from build123d import *

# Parameters (mm, degrees)
BOSS_EXTRUDE1_DEPTH = 3.175
FILLET1_R           = 25.4
SKETCH2_R           = 2.25
CUT_EXTRUDE1_DEPTH  = 94.20730796


with BuildPart() as part:
    # Sketch1 → Boss-Extrude1 (new body)
    with BuildSketch(Plane.XY):
        with BuildLine():
            Line((-14.497184722, -4.405622253), (80.752815278, -4.405622253))
            Line((80.752815278, -4.405622253), (80.752815278, -38.596437465))
            ThreePointArc((80.752815278, -38.596437465), (66.572735919, -34.398241716), (57.985570414, -46.438178872))
            Line((57.985570414, -46.438178872), (-14.497184722, -46.438178872))
            Line((-14.497184722, -46.438178872), (-14.497184722, -4.405622253))
        make_face()
        with BuildLine():
            Line((8.180129042, -20.254648783), (43.838119696, -20.254648783))
            ThreePointArc((43.838119696, -20.254648783), (49.538039085, -25.954568173), (43.838119696, -31.654487563))
            Line((43.838119696, -31.654487563), (8.180129042, -31.654487563))
            ThreePointArc((8.180129042, -31.654487563), (2.480209652, -25.954568173), (8.180129042, -20.254648783))
        make_face(mode=Mode.SUBTRACT)
    extrude(amount=BOSS_EXTRUDE1_DEPTH)

    # Fillet1
    fillet1_edges = [part.edges().sort_by_distance(p)[0] for p in [
        (80.752815278, -4.405622253, 1.5875),
        (-14.497184722, -46.438178872, 1.5875),
    ]]
    fillet(fillet1_edges, radius=FILLET1_R)

    # Sketch2 → Cut-Extrude1 (cut, through all)
    with BuildSketch(Plane(origin=(0, 0, 0), x_dir=(-1, 0, 0), z_dir=(0, 0, -1))):
        with Locations((-50.8, -12.699000033)):
            Circle(SKETCH2_R)
        with Locations((6.35, -12.699000033)):
            Circle(SKETCH2_R)
    extrude(amount=-CUT_EXTRUDE1_DEPTH, mode=Mode.SUBTRACT)


solid = part.part
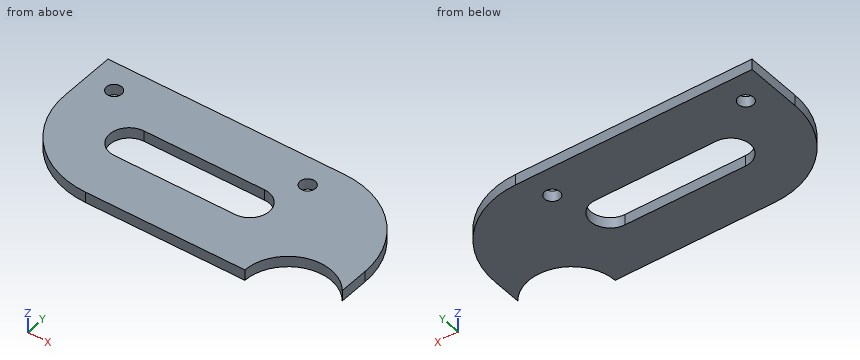
CAD build for the part. Positions are in the model's coordinates, mm. Give positions to 0.01 mm unless a question says otherwise; leave off trailing zeros. Loops run counter-clockwise (first coordinate to the right, second up) from the corner with the lowest first, then second, coordinate; pieces in that order, holes last. Notation, with made-up numbers: M 77.5,-1.5 L 100.5,-1.5 A4 cw 100.5,2.5 Z; hole C -10,88.5 d6. An arc over 180 degrees is marked long. Answer in a Markdown table with one row per item. Add a question column.
Item 1: Band-saw the part on A-A on x = 50.8. Give the cut face in (y, z) (3 decimals).
Item 2: Band-saw the part on B-B on z = 0.8. Give the cut face in (x, y).
Item 3: Drop flat-ended pins along their axis: P1, Ø4, axis at x = 50.8, y = -12.699, coming from the -Z side; P2, Ø6, axis at x = 41, y = -36, coming from the -Z side; P3, Ø1.5, axis at y = -11.5, z = 1, coming from the +X side. Give the stop position or say it passes through.
Item 4: Band-saw the part on C-C on x = -6.35. Give the cut face in (y, z) (3 decimals), then the cut area to 3 significant figures.
Item 5: Probe probe 1 along Y at (x, z) = (10.5, 1.1); probe 2 along Y at (x, z) = (7, 0.75); probe 3 along X at (y, z) = (-29.5, 0.2). List the from-to ranges inside material, lowest first.
Item 6: Band-saw the part on D-D on x = 64. Give the cut face in (y, z) (3 decimals), then the cut area to 3 significant figures.
Reply:
| question | item | result |
|---|---|---|
| 1 | outline | M -46.438,0 L -14.949,0 L -14.949,3.175 L -46.438,3.175 Z; M -10.449,0 L -4.406,0 L -4.406,3.175 L -10.449,3.175 Z |
| 2 | outline | M -14.5,-21.04 A25.4 ccw 10.9,-46.44 L 57.99,-46.44 A12.73 cw 80.75,-38.6 L 80.75,-29.81 A25.4 ccw 55.35,-4.41 L -14.5,-4.41 Z; hole C -6.35,-12.7 d4.5; hole M 8.18,-31.65 L 43.84,-31.65 A5.7 ccw 43.84,-20.25 L 8.18,-20.25 A5.7 ccw Z; hole C 50.8,-12.7 d4.5 |
| 3 | P1 | passes through |
| 3 | P2 | stops at z = 0 |
| 3 | P3 | stops at x = 73.71 |
| 4 | outline | M -39.68,0 L -14.949,0 L -14.949,3.175 L -39.68,3.175 Z; M -10.449,0 L -4.406,0 L -4.406,3.175 L -10.449,3.175 Z |
| 4 | area | 97.7 mm^2 |
| 5 | probe 1 | y = -46.43 to -31.65, -20.25 to -4.41 |
| 5 | probe 2 | y = -46.14 to -31.53, -20.38 to -4.41 |
| 5 | probe 3 | x = -13.05 to 3.72, 48.3 to 80.75 |
| 6 | outline | M -35.621,0 L -5.923,0 L -5.923,3.175 L -35.621,3.175 Z |
| 6 | area | 94.3 mm^2 |
